The drawing under review shows one solid part. Ordinate dimensions are in mm from its lowest x, y, z. A direction names the side the tool comes from. Give positions to 0.01 mm unless a question says otherwise; leave off trailing zeros. Loops run counter-clockwise (first coordinate to the right, second up) from the corner with the lowest first, then second, coordinate; pieces in that order, holes last. Notation, with made-up numbers: (22.5, 48) -> (61.5, 48) arc R22 ccw to (61.5, 58) -> close; hole circle Ø10 at (24, 36). An arc over 180 degrees is marked (long way). Answer in a Markdown table with one row per item. Add a question column.
(1) For the marked faces 1, 2 and 3, list the 3-axis set-ups (+Z, -Z, +X, -X, +Y, -Y) from which the entire face can be reached by the end or side of a thin tool; tool diameter is ignored.
(2) Consider section C-C on y = 2.9. Write out the cut boundary in (x, z) (1 decimal).
(3) For line 1 (Z direction, x = 26.5, y = 0.6); line 2 (X direction, y = 3.45, z = 5.25); line 3 (Y direction, x = 8.5, z = 9.5), list the stretches that pass through material, from the lowest coordinate up.
(4) For pin 1 (1.8 mm diameter, centred on x = 20, y = 5.5, fed in from -Z); pin 2 (0.8 mm diameter, centred on x = 29.5, y = 3, fed in from -Z) (1 decimal); pin 3 (5 mm diameter, centred on x = 28, z = 4.5, fed in from -Y), all flat-tipped, find the tip position at first contact; note any pin that passes through.
(5) Consider section A-A on z = 4. Write out the cut boundary in (x, y).
(6) Consider section D-D on z = 7.75. Write out the cut boundary in (x, y).
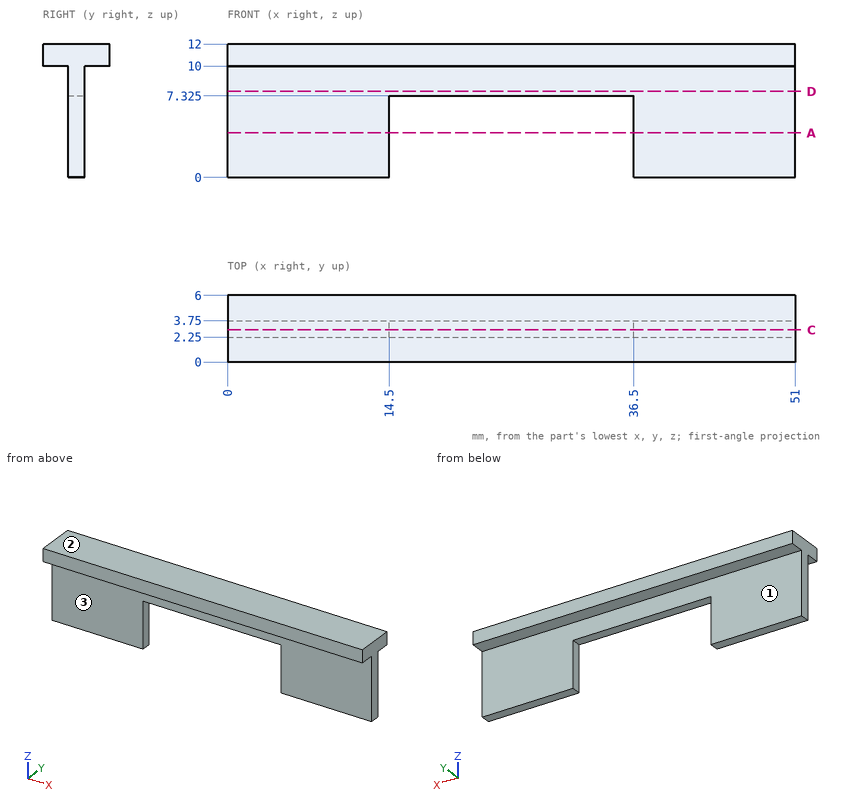
Values follow:
| question | item | result |
|---|---|---|
| 1 | face 1 | -Z, +X, -X, +Y |
| 1 | face 2 | +Z, +X, -X, +Y, -Y |
| 1 | face 3 | -Z, +X, -X, -Y |
| 2 | outline | (0, 0) -> (14.5, 0) -> (14.5, 7.3) -> (36.5, 7.3) -> (36.5, 0) -> (51, 0) -> (51, 12) -> (0, 12) -> close |
| 3 | line 1 | 10 to 12 |
| 3 | line 2 | 0 to 14.5, 36.5 to 51 |
| 3 | line 3 | 2.25 to 3.75 |
| 4 | pin 1 | z = 10 |
| 4 | pin 2 | z = 7.3 |
| 4 | pin 3 | through |
| 5 | outline | (0, 2.25) -> (14.5, 2.25) -> (14.5, 3.75) -> (0, 3.75) -> close; (36.5, 2.25) -> (51, 2.25) -> (51, 3.75) -> (36.5, 3.75) -> close |
| 6 | outline | (0, 2.25) -> (51, 2.25) -> (51, 3.75) -> (0, 3.75) -> close |
